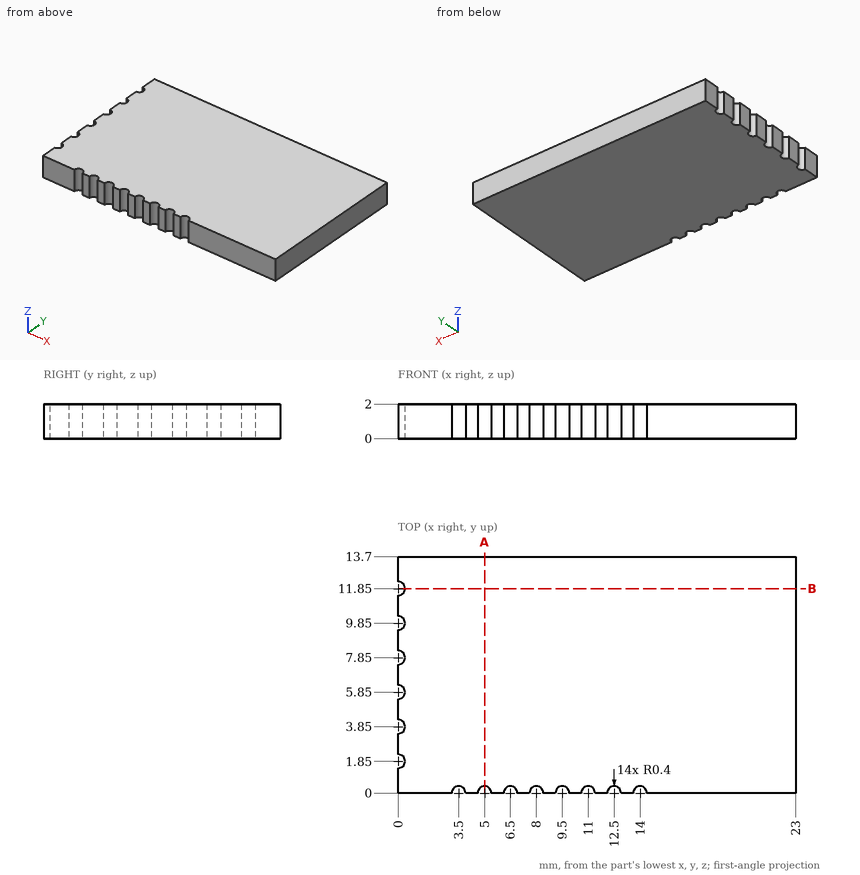
Part print with two shaded views. Sizes in mm from the minimum x, y, z corner. Round coordinates to 2 decimals unless told otherwise and drop trailing zeros. Order: outer loops, then holes, each group sorted by start corner. A loop starts at its lowest first (then second) coordinate and runs counter-clockwise, first axis right, second up. Notation, with made-up numbers: (-1, 0.5) - (24, 0.5) arc R4 ccw to (24, 6.5) - close; hole circle Ø8 at (62, 54). An arc over 180 degrees is marked (long way). Return JSON: item names as keys, results as strings.
(1) Wall check: probe 1 along Y at (x, z) = (14, 0.95); probe 2 along Y at (x, z) = (6.25, 0.7); probe 3 along X at (y, z) = (10, 0.35). Give the ranges that are in metal, low to high. Write a range as from..to.
Answer key:
{"probe 1": "y = 0.4..13.7", "probe 2": "y = 0.31..13.7", "probe 3": "x = 0.37..23"}
(2) Pin check, flat tip, straight feed: pin 1 Ø1 at (x, z) = (15, 0.5) entering from -Y. Stop position of the tip, or through.
Answer key:
{"pin 1": "stops at y = 0"}
(3) Cut at A-A (x = 5). Give the cut face in (y, z).
Answer key:
{"outline": "(0.4, 0) - (13.7, 0) - (13.7, 2) - (0.4, 2) - close"}
(4) Cut at B-B (y = 11.85). Give the cut face in (x, z).
Answer key:
{"outline": "(0.4, 0) - (23, 0) - (23, 2) - (0.4, 2) - close"}
